Can you work these out from the drawing? Everything is in mm from the part's minimum corner. Coordinates: 2 decimals unless noted, no trailing zeros. Loops run counter-clockwise (first coordinate to the right, second up) from the corner with the lowest first, then second, coordinate; pieces in that order, holes last. Notation, with made-up numbers: (-18.5, -3) -> (38.5, -3) arc R24 cw to (38.5, 23) -> close; hole circle Ø4 at (28.25, 51.5). An arc over 180 degrees is marked (long way). Put each result on its own line as item: value. Start each with the question number.
Item 1: If we section it at C-C on y = 4.3: Please give me the cut outline in (x, z), plus the area to 3 significant figures.
Item 2: If we section it at B-B on x = 22: Please give me the cut outline in (y, z).
Item 3: Will these pins go through, and if not, where does the flat tip stop? P1, Ø2.5, axis at x = 22, z = 7, coming from the -Y side; P2, Ø7, axis at x = 32.76, z = 7, coming from the +Y side.
Item 4: If we section it at D-D on x = 14: Please give me the cut outline in (y, z).
Item 5: If we section it at A-A on z = 23: Please give me the cut outline in (x, y).
Item 6: Please list where these lines run through material, in increasing order: L1, parallel to Z at x = 32.76, y = 1.2; L2, parallel to X at y = 0.85, z = 23; L3, parallel to X at y = 1, z = 7.75. Write a range as from..to.
Item 7: We'd pull the mould along Z, two halves only. Please class the marked faces 1, 2, 3 and 4: pulls with the +Z half, pulls with the -Z half, needs draft (parallel to the pull), parting line crosses it, or undercut.
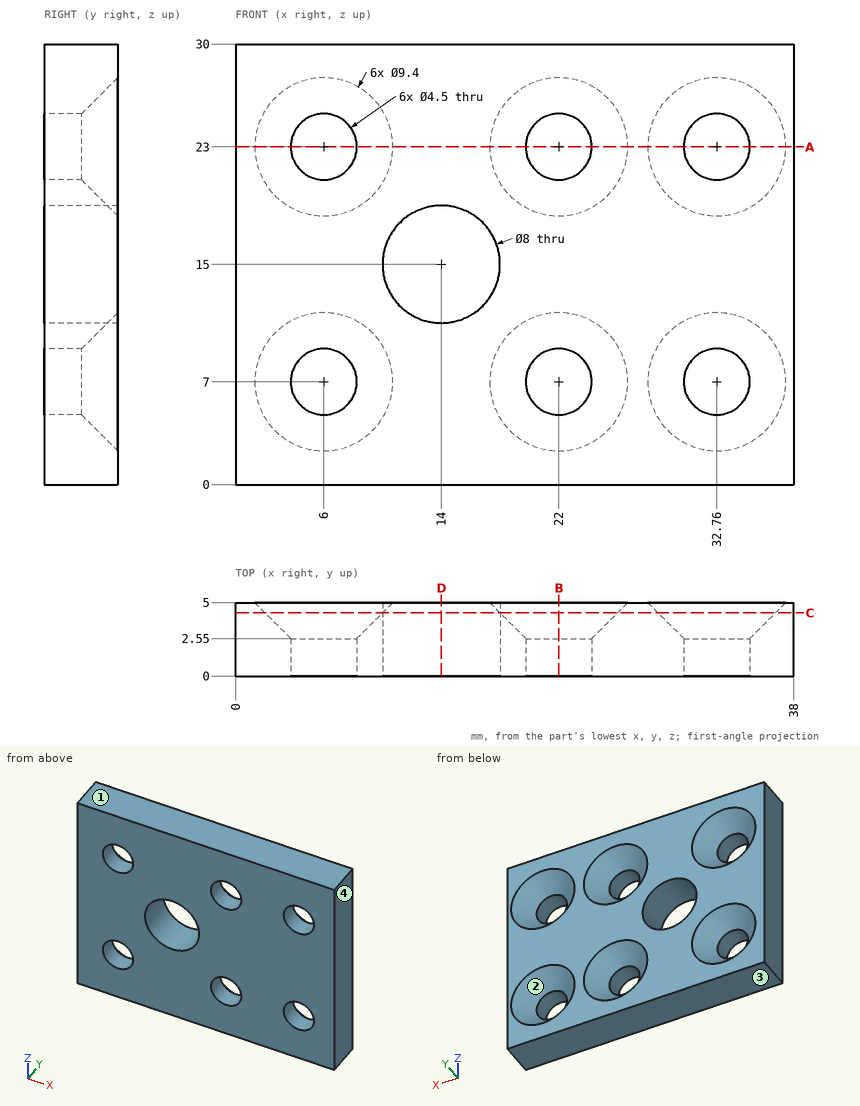
Solutions:
1. outline: (0, 0) -> (38, 0) -> (38, 30) -> (0, 30) -> close; hole circle Ø8 at (6, 7); hole circle Ø8 at (6, 23); hole circle Ø8 at (14, 15); hole circle Ø8 at (22, 7); hole circle Ø8 at (22, 23); hole circle Ø8 at (32.76, 7); hole circle Ø8 at (32.76, 23)
1. area: 788 mm^2
2. outline: (0, 0) -> (5, 0) -> (5, 2.3) -> (2.55, 4.75) -> (0, 4.75) -> close; (0, 9.25) -> (2.55, 9.25) -> (5, 11.7) -> (5, 18.3) -> (2.55, 20.75) -> (0, 20.75) -> close; (0, 25.25) -> (2.55, 25.25) -> (5, 27.7) -> (5, 30) -> (0, 30) -> close
3. P1: through
3. P2: y = 3.8
4. outline: (0, 0) -> (5, 0) -> (5, 11) -> (0, 11) -> close; (0, 19) -> (5, 19) -> (5, 30) -> (0, 30) -> close
5. outline: (0, 0) -> (3.75, 0) -> (3.75, 2.55) -> (1.3, 5) -> (0, 5) -> close; (8.25, 0) -> (19.75, 0) -> (19.75, 2.55) -> (17.3, 5) -> (10.7, 5) -> (8.25, 2.55) -> close; (24.25, 0) -> (30.51, 0) -> (30.51, 2.55) -> (28.06, 5) -> (26.7, 5) -> (24.25, 2.55) -> close; (35.01, 0) -> (38, 0) -> (38, 5) -> (37.46, 5) -> (35.01, 2.55) -> close
6. L1: 0..4.75, 9.25..20.75, 25.25..30
6. L2: 0..3.75, 8.25..19.75, 24.25..30.51, 35.01..38
6. L3: 0..3.88, 8.12..19.88, 24.12..30.64, 34.88..38
7. face 1: pulls with the +Z half
7. face 2: undercut
7. face 3: pulls with the -Z half
7. face 4: needs draft
